```python
from build123d import *

# Parameters (mm, degrees)
SKETCH1_W           = 127
SKETCH1_H           = 76.2
BOSS_EXTRUDE1_DEPTH = 6.35
SKETCH2_R           = 3.175
SKETCH2_R_2         = 9.525
CUT_EXTRUDE1_DEPTH  = 75.324844433


with BuildPart() as part:
    # Sketch1 → Boss-Extrude1 (new body)
    with BuildSketch(Plane(origin=(0, 0, 0), x_dir=(1, 0, 0), z_dir=(0, 1, 0))):
        Rectangle(SKETCH1_W, SKETCH1_H)
    extrude(amount=BOSS_EXTRUDE1_DEPTH)

    # Sketch2 → Cut-Extrude1 (cut, through all)
    with BuildSketch(Plane(origin=(0, 6.35, 0), x_dir=(1, 0, 0), z_dir=(0, 1, 0))):
        with Locations(Location((-41.275, 28.575, 0), (0, 0, 270))):
            Circle(SKETCH2_R)
        with Locations(Location((41.275, 28.575, 0), (0, 0, 270))):
            Circle(SKETCH2_R)
        with Locations(Location((41.275, -28.575, 0), (0, 0, 270))):
            Circle(SKETCH2_R)
        with Locations(Location((-41.275, -28.575, 0), (0, 0, 270))):
            Circle(SKETCH2_R)
        with Locations(Location((-19.05, 19.05, 0), (0, 0, 270))):
            Circle(SKETCH2_R)
        with Locations(Location((19.05, 19.05, 0), (0, 0, 270))):
            Circle(SKETCH2_R)
        with Locations(Location((19.05, -19.05, 0), (0, 0, 270))):
            Circle(SKETCH2_R)
        with Locations(Location((-19.05, -19.05, 0), (0, 0, 270))):
            Circle(SKETCH2_R)
        with Locations(Location((0, 0, 0), (0, 0, 270))):
            Circle(SKETCH2_R_2)
    extrude(amount=-CUT_EXTRUDE1_DEPTH, mode=Mode.SUBTRACT)


solid = part.part
```
Input: part model. Units: mm. Frame: model coordinates. Coordinates: 2 decimals unless noted, no trailing zeros. Order: outer loops, then holes, each group sorted by start corner. A loop starts at its lowest first (then second) coordinate and runs counter-clockwise, first axis right, second up. Notation, with made-up numbers: (1.25, 15.25) - (29.25, 15.25) arc R11 ccw to (29.25, 19.25) - close; hole circle Ø1 at (68.5, 31.25). An arc over 180 degrees is marked (long way). Return JSON: item names as keys, results as strings.
Q1. Ray query, probe 1 along X at (y, z) = (3, -19.05) (3 decimals); probe 2 along Z at (x, y) = (-21, 3.25); probe 3 along X at (y, z) = (4, 0) (3 decimals). Return the intervals inside material, ascending.
The answers:
{"probe 1": "x = -63.5 to -22.225, -15.875 to 15.875, 22.225 to 63.5", "probe 2": "z = -38.1 to -21.56, -16.54 to 16.54, 21.56 to 38.1", "probe 3": "x = -63.5 to -9.525, 9.525 to 63.5"}
Q2. First-contact query: pin 1 (7.5 mm diameter, centred on x = -19.05, z = -19.05, fed in from +Y). Flat tip, straight axial feed; report the tip coordinate or a pass-through.
The answers:
{"pin 1": "stops at y = 6.35"}
Q3. Cut plane D-D (z = 19.05). Return loops of the section in (x, y) (3 decimals).
The answers:
{"outline": "(-63.5, 0) - (-22.225, 0) - (-22.225, 6.35) - (-63.5, 6.35) - close; (-15.875, 0) - (15.875, 0) - (15.875, 6.35) - (-15.875, 6.35) - close; (22.225, 0) - (63.5, 0) - (63.5, 6.35) - (22.225, 6.35) - close"}
Q4. Cut plane A-A (z = 0). Return loops of the section in (x, y) (3 decimals), then the cut area to 3 significant figures.
The answers:
{"outline": "(-63.5, 0) - (-9.525, 0) - (-9.525, 6.35) - (-63.5, 6.35) - close; (9.525, 0) - (63.5, 0) - (63.5, 6.35) - (9.525, 6.35) - close", "area": "685 mm2"}
Q5. Draft query along Z for faces 1 (the flat face through (63.5, 3, 1)), 2 (the flat face through (-1, 3, 38.1)), 3 (the cylindrical face through (-43.2, 3.2, -31.1)). Return one class per face: +Z half, -Z half, draft (parallel to the pull), parting line (faces both ways), or undercut.
The answers:
{"face 1": "draft", "face 2": "+Z half", "face 3": "undercut"}
Q6. Cut plane B-B (x = -19.05). Return loops of the section in (y, z) (3 decimals).
The answers:
{"outline": "(0, -38.1) - (6.35, -38.1) - (6.35, -22.225) - (0, -22.225) - close; (0, -15.875) - (6.35, -15.875) - (6.35, 15.875) - (0, 15.875) - close; (0, 22.225) - (6.35, 22.225) - (6.35, 38.1) - (0, 38.1) - close"}
Q7. Cut plane C-C (x = 0). Return loops of the section in (y, z) (3 decimals).
The answers:
{"outline": "(0, -38.1) - (6.35, -38.1) - (6.35, -9.525) - (0, -9.525) - close; (0, 9.525) - (6.35, 9.525) - (6.35, 38.1) - (0, 38.1) - close"}
